```python
from build123d import *

# Parameters (mm, degrees)
SKETCH1_R            = 17.4625
SKETCH1_R_2          = 12.7
SPRING_CHAMBER_DEPTH = 28.575
BALL_CHAMBER_START   = 47.625
SKETCH2_R            = 17.4625
SKETCH2_R_2          = 9.525
BALL_CHAMBER_DEPTH   = 47.625
SKETCH5_R            = 3.81
BALL_HOLE_DEPTH      = 54.647166165
SKETCH8_R            = 17.4625
SKETCH8_R_2          = 11.90625
CUT_EXTRUDE2_DEPTH   = 41.275
SKETCH6_R            = 17.4625
SKETCH6_R_2          = 1.651
BOSS_EXTRUDE4_DEPTH  = 6.35


with BuildPart() as part:
    # Sketch1 → spring_chamber (new body)
    with BuildSketch(Plane(origin=(0, 0, 0), x_dir=(1, 0, 0), z_dir=(0, 1, 0))):
        with Locations(Location((0, 0, 0), (0, 0, 270))):
            Circle(SKETCH1_R)
        with Locations(Location((0, 0, 0), (0, 0, 270))):
            Circle(SKETCH1_R_2, mode=Mode.SUBTRACT)
    extrude(amount=SPRING_CHAMBER_DEPTH)

    # Sketch2 → ball_chamber (add)
    with BuildSketch(Plane.XZ.offset(BALL_CHAMBER_START)):
        with Locations(Location((0, 0, 0), (0, 0, 270))):
            Circle(SKETCH2_R)
        with Locations(Location((0, 0, 0), (0, 0, 270))):
            Circle(SKETCH2_R_2, mode=Mode.SUBTRACT)
    extrude(amount=-BALL_CHAMBER_DEPTH)

    # Sketch5 → ball_hole (cut, through all)
    with BuildSketch(Plane(origin=(0, 0, 0), x_dir=(0, 0, -1), z_dir=(1, 0, 0))):
        with Locations(Location((0, -25.4, 0), (0, 0, 180))):
            Circle(SKETCH5_R)
    ball_hole = extrude(amount=BALL_HOLE_DEPTH, mode=Mode.SUBTRACT)

    # Sketch8 → Cut-Extrude2 (cut)
    with BuildSketch(Plane.XZ.offset(47.625)):
        with Locations(Location((0, 0, 0), (0, 0, 270))):
            Circle(SKETCH8_R)
        with Locations(Location((0, 0, 0), (0, 0, 270))):
            Circle(SKETCH8_R_2, mode=Mode.SUBTRACT)
    extrude(amount=-CUT_EXTRUDE2_DEPTH, mode=Mode.SUBTRACT)

    # Mirror1: ball_hole across plane
    add(ball_hole.mirror(Plane(origin=(0, 0, 0), x_dir=(0, 0, 1), z_dir=(1, 0, 0))), mode=Mode.SUBTRACT)

    # Sketch6 → Boss-Extrude4 (add)
    with BuildSketch(Plane(origin=(0, 28.575, 0), x_dir=(1, 0, 0), z_dir=(0, 1, 0))):
        with BuildLine():
            ThreePointArc((-28.810185185, 6.345643224), (-34.925, 0), (-28.810185185, -6.345643224))
            ThreePointArc((-28.810185185, -6.345643224), (-23.017865483, -7.988458599), (-18.633080808, -12.114409792))
            ThreePointArc((-18.633080808, -12.114409792), (0, -22.225), (18.633080808, -12.114409792))
            ThreePointArc((18.633080808, -12.114409792), (23.017865483, -7.988458599), (28.810185185, -6.345643224))
            ThreePointArc((28.810185185, -6.345643224), (34.925, 0), (28.810185185, 6.345643224))
            ThreePointArc((28.810185185, 6.345643224), (23.017865483, 7.988458599), (18.633080808, 12.114409792))
            ThreePointArc((18.633080808, 12.114409792), (0, 22.225), (-18.633080808, 12.114409792))
            ThreePointArc((-18.633080808, 12.114409792), (-23.017865483, 7.988458599), (-28.810185185, 6.345643224))
        make_face()
        with Locations(Location((0, 0, 0), (0, 0, 90))):
            Circle(SKETCH6_R, mode=Mode.SUBTRACT)
        with Locations((-28.575, 0)):
            Circle(SKETCH6_R_2, mode=Mode.SUBTRACT)
        with Locations((28.575, 0)):
            Circle(SKETCH6_R_2, mode=Mode.SUBTRACT)
    extrude(amount=BOSS_EXTRUDE4_DEPTH)


with BuildPart() as boss_extrude4_kept_piece:
    # of the separate pieces the step leaves, the one the design keeps (boss_extrude4_pieces_kept)
    add(part.part.solids().sort_by_distance((0, 0, 17.4625))[0])


solid = boss_extrude4_kept_piece.part
```
The listing builds one solid part. Answer for the finished solid, in the listing's coordinates (mm). A direction names the side the tool comes from. Coordinates: 2 decimals unless noted, no trailing zeros. Write each loop counter-clockwise with the first axis right and the second up, starting at its lowest first coordinate (ties: lowest second). Pieces come first, ordered by that corner, then holes. Notation, with made-up numbers: (47, 55) - (63, 55) arc R22 cw to (63, 86) - close; hole circle Ø3 at (-15, -8). An arc over 180 degrees is marked (long way). One line per item, written item: value.
1) Consider line 1 along X through (y, z) = (17, 0); line 2 along Y through (x, z) = (-9.8, 0) (3 decimals); line 3 along X through (y, z) = (-14, 0) (3 decimals). Determine where each line is inside the solid, lowest interval first. Write a range as from..to.
Geometry check:
line 1: x = -17.46..-12.7, 12.7..17.46
line 2: y = -47.625..-29.21, -21.59..0
line 3: x = -11.906..-9.525, 9.525..11.906
2) For a pull along Y with two mould halves and no side action, classify faces 1 (the flat face through (9, 0, -5)), 2 (the flat face through (10, -47.625, 0)), 3 (the cylindrical face through (10.31, -21.68, -0.83)) as pulls with the +Y half, pulls with the -Y half, needs draft (parallel to the pull), parting line crosses it, or undercut.
Geometry check:
face 1: pulls with the +Y half
face 2: pulls with the -Y half
face 3: undercut
3) A tool of negligible diameter and unlimited length cuts with its end or side. For faces 4 (the cylindrical face through (-10.31, -21.68, -0.83)), 5 (the cylindrical face through (-7.7, 14.1, -10.1)), 6 (the cylindrical face through (-4.56, -27.28, -11)), from which of +Z, -Z, +X, -X, +Y, -Y can it reach the whole face along a straight path? Write none if from no direction.
Geometry check:
face 4: +X, -X
face 5: +Y
face 6: -Y
4) Find section D-D (z = 8). Give the vertices of the cut face in (x, y) (3 decimals), and give its area (3 significant figures).
Geometry check:
outline: (-15.522, -6.35) - (-8.818, -6.35) - (-8.818, -47.625) - (-5.17, -47.625) - (-5.17, 0) - (-9.864, 0) - (-9.864, 28.575) - (-15.522, 28.575) - close; (5.17, -47.625) - (8.818, -47.625) - (8.818, -6.35) - (15.522, -6.35) - (15.522, 28.575) - (9.864, 28.575) - (9.864, 0) - (5.17, 0) - close
area: 756 mm2
5) Find section B-B (z = 0). Count the separate pieces of the cut face and the enclosed holes in it, and give its area (3 significant figures).
Geometry check:
separate pieces: 4
enclosed holes: 0
area: 533 mm2
6) Each of these flat-tipped pins is pushed along its axis until it touches: pin 1 Ø9 at (y, z) = (-25.4, 0) entering from -X; pin 2 Ø5 at (x, y) = (4, 19) entering from -Z; pin 3 Ø10 at (y, z) = (-25.4, 0) entering from +X; pin 4 Ø2 at (x, z) = (6.5, 4.5) entering from +Y. Where does it stop, or does it pass through?
Geometry check:
pin 1: stops at x = -11.91
pin 2: stops at z = -17.4
pin 3: stops at x = 11.91
pin 4: passes through
